```python
from build123d import *

# Parameters (mm, degrees)
SKETCH_2_R      = 1.8
EXTRUDE_1_DEPTH = 3


with BuildPart() as part:
    # 草图2 → 凸台-拉伸1 (new body)
    with BuildSketch(Plane.XY):
        with BuildLine():
            Line((0, 0), (-5, 0))
            Line((-5, 0), (-5, -5))
            Line((-5, -5), (0, -5))
            ThreePointArc((0, -5), (2.5, -2.5), (0, 0))
        make_face()
        with Locations((0, -2.5)):
            Circle(SKETCH_2_R, mode=Mode.SUBTRACT)
    extrude(amount=EXTRUDE_1_DEPTH)


solid = part.part
```
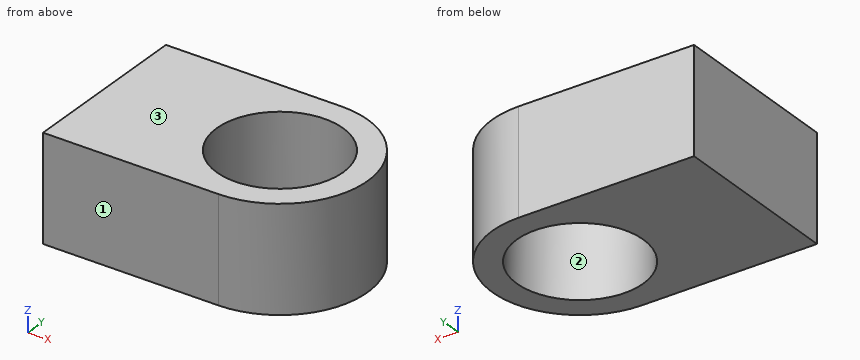
CAD build for the part. Positions are in the model's coordinates, mm. Face numbers are marked on the shaded views. Coordinates: 2 decimals unless noted, no trailing zeros. Order: outer loops, then holes, each group sorted by start corner. A loop starts at its lowest first (then second) coordinate and runs counter-clockwise, first axis right, second up. Notation, with made-up numbers: (-9.75, 36.25) - (29.25, 36.25) arc R6 ccw to (29.25, 45.25) - close; hole circle Ø10 at (-36.5, 76.5). An arc over 180 degrees is marked (long way). Use a Markdown table: item, result. Add a question column.
(1) Pull direction Y, two halves, no side cores. Call the marked faces 1, 2 and 3: +Y half, -Y half, draft (parallel to the pull), parting line (faces both ways), or undercut.
(2) Flat gauge pin, fed straight in: pin 1 (1 mm diameter, centred on x = -0.5, y = -3, fed in from -Z). Where does the tip first touch, or does it go through?
(3) Saw through at A-A (y = -2.5). Give the cut face in (x, z), then the cut area to 3 significant figures.
(4) Saw through at D-D (y = -0.6). Give the cut face in (x, z), then the cut area to 3 significant figures.
(5) Saw through at C-C (z = 1.55). Give the cut face in (x, y).
(6) Drill centre lines: line 1 along X through (y, z) = (-1.4, 0.6) (3 decimals); line 2 along Y through (x, z) = (-0.75, 2.05); line 3 along X through (y, z) = (-0.9, 1.8). Where is each one in solid material? Low to high. Write a range as [from, to].
(7) Saw through at B-B (x = 1.5). Give the cut face in (y, z), then the cut area to 3 significant figures.
Solved:
| question | item | result |
|---|---|---|
| 1 | face 1 | -Y half |
| 1 | face 2 | undercut |
| 1 | face 3 | draft |
| 2 | pin 1 | passes through |
| 3 | outline | (-5, 0) - (-1.8, 0) - (-1.8, 3) - (-5, 3) - close; (1.8, 0) - (2.5, 0) - (2.5, 3) - (1.8, 3) - close |
| 3 | area | 11.7 mm² |
| 4 | outline | (-5, 0) - (1.62, 0) - (1.62, 3) - (-5, 3) - close |
| 4 | area | 19.9 mm² |
| 5 | outline | (-5, -5) - (0, -5) arc R2.5 ccw to (0, 0) - (-5, 0) - close; hole circle Ø3.6 at (0, -2.5) |
| 6 | line 1 | x = [-5, -1.425], [1.425, 2.245] |
| 6 | line 2 | y = [-5, -4.14], [-0.86, 0] |
| 6 | line 3 | x = [-5, -0.82], [0.82, 1.92] |
| 7 | outline | (-4.5, 0) - (-3.49, 0) - (-3.49, 3) - (-4.5, 3) - close; (-1.51, 0) - (-0.5, 0) - (-0.5, 3) - (-1.51, 3) - close |
| 7 | area | 6.03 mm² |
